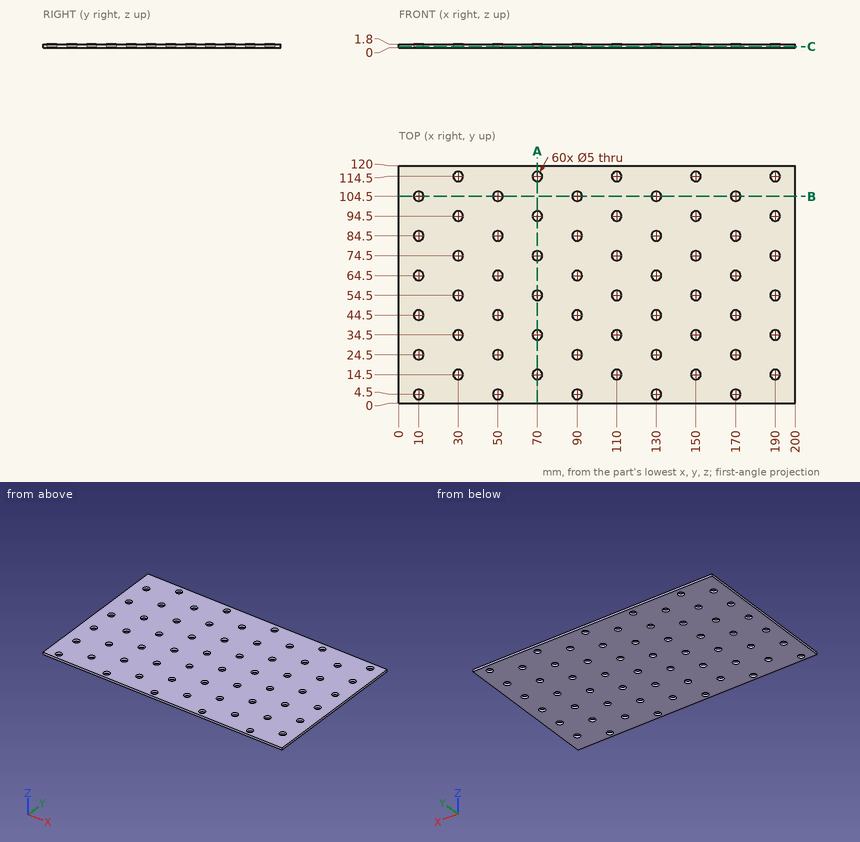
Check sheet for the drawn part. Datum: minimum x, y, z corner. Units: mm. Round coordinates to 2 decimals unless told otherwise and drop trailing zeros. Order: outer loops, then holes, each group sorted by start corner. A loop starts at its lowest first (then second) coordinate and runs counter-clockwise, first axis right, second up.
(1) Cross-section at C-C, the plane z = 0.5. State how many separate pieces and enclosed holes the cut face has, and give its area (3 significant figures).
(2) Cross-section at A-A, the plane x = 70. Enter the section's corners in (y, z).
(3) Go/stop test with flat-tipped pins: P1, Ø4, axis at x = 30, y = 94.5, coming from the -Z side; P2, Ø3, axis at x = 100, y = 101, coming from the -Z side. Record where each tip stops, or that it passes through.
(4) Cross-section at B-B, the plane y = 104.5. Enter the section's corners in (x, z).
(5) Scan lines: probe 1 along X at (y, z) = (113, 0.8); probe 2 along X at (y, z) = (86, 1.7). Record each from-to range of solid material in increasing order.
Check sheet entries:
1. separate pieces: 1
1. enclosed holes: 60
1. area: 22,800 mm2
2. outline: (0, 0) - (12, 0) - (12, 1.8) - (0, 1.8) - close; (17, 0) - (32, 0) - (32, 1.8) - (17, 1.8) - close; (37, 0) - (52, 0) - (52, 1.8) - (37, 1.8) - close; (57, 0) - (72, 0) - (72, 1.8) - (57, 1.8) - close; (77, 0) - (92, 0) - (92, 1.8) - (77, 1.8) - close; (97, 0) - (112, 0) - (112, 1.8) - (97, 1.8) - close; (117, 0) - (120, 0) - (120, 1.8) - (117, 1.8) - close
3. P1: passes through
3. P2: stops at z = 0
4. outline: (0, 0) - (7.5, 0) - (7.5, 1.8) - (0, 1.8) - close; (12.5, 0) - (47.5, 0) - (47.5, 1.8) - (12.5, 1.8) - close; (52.5, 0) - (87.5, 0) - (87.5, 1.8) - (52.5, 1.8) - close; (92.5, 0) - (127.5, 0) - (127.5, 1.8) - (92.5, 1.8) - close; (132.5, 0) - (167.5, 0) - (167.5, 1.8) - (132.5, 1.8) - close; (172.5, 0) - (200, 0) - (200, 1.8) - (172.5, 1.8) - close
5. probe 1: x = 0 to 28, 32 to 68, 72 to 108, 112 to 148, 152 to 188, 192 to 200
5. probe 2: x = 0 to 8, 12 to 48, 52 to 88, 92 to 128, 132 to 168, 172 to 200
